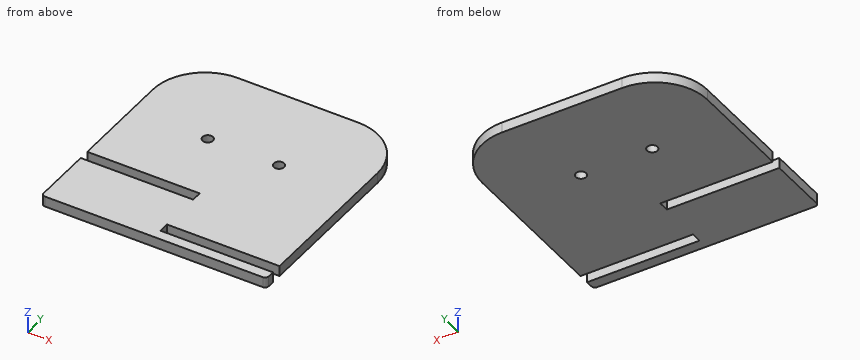
from build123d import *

# Parameters (mm, degrees)
BOSS_EXTRUDE7_DEPTH = 3
SKETCH3_R           = 1.5
CUT_EXTRUDE1_DEPTH  = 3


with BuildPart() as part:
    # Sketch1 → Boss-Extrude7 (new body)
    with BuildSketch(Plane.XY):
        with BuildLine():
            Line((-46.661503554, -6.485084804), (-12.261503554, -6.485084804))
            ThreePointArc((-12.261503554, -6.485084804), (-1.654901836, -10.878483086), (2.738496446, -21.485084804))
            Line((2.738496446, -21.485084804), (2.738496446, -66.485084804))
            Line((2.738496446, -66.485084804), (-29.461503554, -66.485084804))
            Line((-29.461503554, -66.485084804), (-29.461503554, -69.485084804))
            Line((-29.461503554, -69.485084804), (2.738496446, -69.485084804))
            Line((2.738496446, -69.485084804), (2.738496446, -71.485084804))
            ThreePointArc((2.738496446, -71.485084804), (2.445603227, -72.192191585), (1.738496446, -72.485084804))
            Line((1.738496446, -72.485084804), (-60.661503554, -72.485084804))
            ThreePointArc((-60.661503554, -72.485084804), (-61.368610335, -72.192191585), (-61.661503554, -71.485084804))
            Line((-61.661503554, -71.485084804), (-61.661503554, -54.485084804))
            Line((-61.661503554, -54.485084804), (-29.461503554, -54.485084804))
            Line((-29.461503554, -54.485084804), (-29.461503554, -51.485084804))
            Line((-29.461503554, -51.485084804), (-61.661503554, -51.485084804))
            Line((-61.661503554, -51.485084804), (-61.661503554, -21.485084804))
            ThreePointArc((-61.661503554, -21.485084804), (-57.268105272, -10.878483086), (-46.661503554, -6.485084804))
        make_face()
    extrude(amount=BOSS_EXTRUDE7_DEPTH)

    # Sketch3 → Cut-Extrude1 (cut)
    with BuildSketch(Plane.XY.offset(3)):
        with Locations((-19.261503554, -31.485084804)):
            Circle(SKETCH3_R)
        with Locations((-39.661503554, -31.485084804)):
            Circle(SKETCH3_R)
    extrude(amount=-CUT_EXTRUDE1_DEPTH, mode=Mode.SUBTRACT)


solid = part.part
Can you work these out from the model? Positions are in its coordinate system, mm. Give positions to 0.01 mm unless a question says otherwise; leave off trailing zeros. Order: outer loops, then holes, each group sorted by start corner. A loop starts at its lowest first (then second) coordinate and runs counter-clockwise, first axis right, second up. Notation, with made-up numbers: M 19.5,42 L 67.5,42 A24 ccw 67.5,55 Z; hole C 8.25,84.25 d10. An arc over 180 degrees is marked long. Use one line per item in the form item = value. Start each with the question number.
Item 1: If I drill on line 1 along Y through (x, z) = (-15, 1.5); line 2 along Y through (x, z) = (-46.5, 2.4); line 3 along X through (y, z) = (-13, 1.95), over which ranges is the centre line in solid material (lowest first)?
Item 2: If we section it at B-B (z = 1.25): Write out the boundary of the cut face in (x, y), then the cut area to 3 significant figures.
Item 3: If we section it at C-C (x = -9.5): Write out the boundary of the cut face in (y, z), then the cut area to 3 significant figures.
Item 4: If we section it at A-A (x = -37): Write out the boundary of the cut face in (y, z).
Item 5: Will these pins go through, and if not, where does the flat tip stop? pin 1 Ø1.5 at (y, z) = (-53, 1.5) entering from -X; pin 2 Ø0.9 at (y, z) = (-68, 1.5) entering from +X.
Outcome:
q1.line_1 = -72.49 to -69.49, -66.49 to -6.49
q1.line_2 = -72.49 to -54.49, -51.49 to -6.49
q1.line_3 = -59.03 to 0.11
q2.outline = M -61.66,-71.49 A1 ccw -60.66,-72.49 L 1.74,-72.49 A1 ccw 2.74,-71.49 L 2.74,-69.49 L -29.46,-69.49 L -29.46,-66.49 L 2.74,-66.49 L 2.74,-21.49 A15 ccw -12.26,-6.49 L -46.66,-6.49 A15 ccw -61.66,-21.49 L -61.66,-51.49 L -29.46,-51.49 L -29.46,-54.49 L -61.66,-54.49 Z; hole C -39.66,-31.49 d3; hole C -19.26,-31.49 d3
q2.area = 3,950 mm2
q3.outline = M -72.49,0 L -69.49,0 L -69.49,3 L -72.49,3 Z; M -66.49,0 L -6.74,0 L -6.74,3 L -66.49,3 Z
q3.area = 188 mm2
q4.outline = M -72.49,0 L -54.49,0 L -54.49,3 L -72.49,3 Z; M -51.49,0 L -6.49,0 L -6.49,3 L -51.49,3 Z
q5.pin_1 = -29.46
q5.pin_2 = -29.46
